```python
from build123d import *

# Parameters (mm, degrees)
BOSS_EXTRUDE1_DEPTH      = 162.5
BOSS_EXTRUDE2_DEPTH      = 43.5
BOSS_EXTRUDE2_DEPTH_BACK = 145
SKETCH3_R                = 81.25
CUT_EXTRUDE1_DEPTH       = 150
SKETCH6_R                = 87.5
SKETCH6_R_2              = 81.25
BOSS_EXTRUDE4_DEPTH      = 43.5
SKETCH7_R                = 115.75
BOSS_EXTRUDE5_DEPTH      = 12.5
SKETCH8_R                = 7.5
CUT_EXTRUDE2_DEPTH       = 12.5
CUT_EXTRUDE3_DEPTH       = 315.329842681
CUT_EXTRUDE3_DEPTH_BACK  = 315.329842681
SKETCH9_R                = 18.75


with BuildPart() as part:
    # Sketch1 → Boss-Extrude1 (new body)
    with BuildSketch(Plane.XY):
        with BuildLine():
            Line((-150, -169), (150, -169))
            Line((150, -169), (82.827141263, 28.211959701))
            ThreePointArc((82.827141263, 28.211959701), (0, 87.5), (-82.827141263, 28.211959701))
            Line((-82.827141263, 28.211959701), (-150, -169))
        make_face()
    extrude(amount=BOSS_EXTRUDE1_DEPTH)

    # Sketch2 → Boss-Extrude2 (add, two sides: drawn at the far end of the back side and taken through both)
    with BuildSketch(Plane.XY.offset(162.5).offset(-BOSS_EXTRUDE2_DEPTH_BACK)):
        with BuildLine():
            Line((-106.53243077, 150), (106.53243077, 150))
            Line((106.53243077, 150), (106.53243077, 135))
            Line((106.53243077, 135), (91.53243077, 135))
            Line((91.53243077, 135), (91.53243077, 120))
            Line((91.53243077, 120), (106.53243077, 120))
            Line((106.53243077, 120), (106.53243077, 105))
            Line((106.53243077, 105), (91.53243077, 105))
            Line((91.53243077, 105), (91.53243077, 90))
            Line((91.53243077, 90), (106.53243077, 90))
            Line((106.53243077, 90), (106.53243077, 75))
            Line((106.53243077, 75), (91.53243077, 75))
            Line((91.53243077, 75), (91.53243077, 60))
            Line((91.53243077, 60), (106.53243077, 60))
            Line((106.53243077, 60), (106.53243077, 45))
            Line((106.53243077, 45), (91.53243077, 45))
            Line((91.53243077, 45), (91.53243077, 30))
            Line((91.53243077, 30), (106.53243077, 30))
            Line((106.53243077, 30), (106.53243077, -41.384104643))
            Line((106.53243077, -41.384104643), (82.827141263, 28.211959701))
            ThreePointArc((82.827141263, 28.211959701), (0, 87.5), (-82.827141263, 28.211959701))
            Line((-82.827141263, 28.211959701), (-106.53243077, -41.384104643))
            Line((-106.53243077, -41.384104643), (-106.53243077, 30))
            Line((-106.53243077, 30), (-91.53243077, 30))
            Line((-91.53243077, 30), (-91.53243077, 45))
            Line((-91.53243077, 45), (-106.53243077, 45))
            Line((-106.53243077, 45), (-106.53243077, 60))
            Line((-106.53243077, 60), (-91.53243077, 60))
            Line((-91.53243077, 60), (-91.53243077, 75))
            Line((-91.53243077, 75), (-106.53243077, 75))
            Line((-106.53243077, 75), (-106.53243077, 90))
            Line((-106.53243077, 90), (-91.53243077, 90))
            Line((-91.53243077, 90), (-91.53243077, 105))
            Line((-91.53243077, 105), (-106.53243077, 105))
            Line((-106.53243077, 105), (-106.53243077, 120))
            Line((-106.53243077, 120), (-91.53243077, 120))
            Line((-91.53243077, 120), (-91.53243077, 135))
            Line((-91.53243077, 135), (-106.53243077, 135))
            Line((-106.53243077, 135), (-106.53243077, 150))
        make_face()
    extrude(amount=BOSS_EXTRUDE2_DEPTH + BOSS_EXTRUDE2_DEPTH_BACK)

    # Sketch3 → Cut-Extrude1 (cut)
    with BuildSketch(Plane.XY.offset(162.5)):
        Circle(SKETCH3_R)
    extrude(amount=-CUT_EXTRUDE1_DEPTH, mode=Mode.SUBTRACT)

    # Sketch6 → Boss-Extrude4 (add, through all)
    with BuildSketch(Plane.XY.offset(162.5)):
        Circle(SKETCH6_R)
        Circle(SKETCH6_R_2, mode=Mode.SUBTRACT)
    extrude(amount=BOSS_EXTRUDE4_DEPTH)

    # Sketch7 → Boss-Extrude5 (add)
    with BuildSketch(Plane.XY.offset(206)):
        with Locations(Location((0, 0, 0), (0, 0, 156.979731296))):
            Circle(SKETCH7_R)
    extrude(amount=BOSS_EXTRUDE5_DEPTH)

    # Sketch8 → Cut-Extrude2 (cut)
    with BuildSketch(Plane.XY.offset(218.5)):
        with Locations((0, -106.25)):
            Circle(SKETCH8_R)
        with Locations((-92.015199152, 53.125)):
            Circle(SKETCH8_R)
        with Locations((92.015199152, 53.125)):
            Circle(SKETCH8_R)
    extrude(amount=-CUT_EXTRUDE2_DEPTH, mode=Mode.SUBTRACT)

    # Sketch9 → Cut-Extrude3 (cut, two sides: drawn at the far end of the back side and taken through both)
    with BuildSketch(Plane.XY.offset(218.5).offset(-CUT_EXTRUDE3_DEPTH_BACK)):
        Circle(SKETCH9_R)
    extrude(amount=CUT_EXTRUDE3_DEPTH + CUT_EXTRUDE3_DEPTH_BACK, mode=Mode.SUBTRACT)


solid = part.part
```
CAD build for the part. Positions are in the model's coordinates, mm. A direction names the side the tool comes from. Round coordinates to 2 decimals unless told otherwise and drop trailing zeros. Loops run counter-clockwise (first coordinate to the right, second up) from the corner with the lowest first, then second, coordinate; pieces in that order, holes last. Notation, with made-up numbers: (9, 49.5) - (20, 49.5) arc R14 ccw to (20, 60.5) - close; hole circle Ø8 at (76, 48). An arc over 180 degrees is marked (long way). Return JSON: item names as keys, results as strings. Group by question number.
Q1. Band-saw the part on C-C on y = -106.25. Give the cut face in (x, z).
Q2. Band-saw the part on B-B on y = 0. Give the number of separate pieces and of enclosed holes in the cut face, plus the area to 3 significant figures.
Q3. Band-saw the part on A-A on x = 0. Give the cut face in (y, z).
Q4. Flat gauge pins, fed straight in: pin 1 Ø2 at (y, z) = (54, 27.5) entering from -X; pin 2 Ø12 at (y, z) = (116, 80.5) entering from +X; pin 3 Ø12 at (x, y) = (0, -106.25) entering from +Z. Where does each tip first touch, or does it go through?
Q5. Band-saw the part on D-D on y = 109.5. Give the cut face in (x, z).
Q6. Drill centre lines: line 1 along Y through (x, z) = (0, 215); line 2 along Y through (x, z) = (-102, 154); line 3 along Y through (x, z) = (0, 9.5). Where is each one in solid material? Low to high. Write a range as [from, to].
Q7. Tool access for faces 1 (the face through (99, 75, 110)), 2 (the face through (84.522, 53.455, 212.338)), 3 (the face through (-106.532, 112, 110)), 4 (the face through (106.532, -5, 110)): list every direction of +Z, -Z, +X, -X, +Y, -Y with a clear straight run to the whole face (end or side of a thin tool).
Q8. Two-plate mould, pull along Y, no slides. Class faces 5 (the face through (99, 135, 110)), 6 (the face through (-2, -169, 80)), 7 (the face through (-106.532, 142, 110)): +Y half, -Y half, draft (parallel to the pull), parting line (faces both ways), or undercut.
Solutions:
{
 "1": {"outline": "(-128.63, 0) - (128.63, 0) - (128.63, 162.5) - (-128.63, 162.5) - close; (-45.92, 206) - (-7.5, 206) - (-7.5, 218.5) - (-45.92, 218.5) - close; (7.5, 206) - (45.92, 206) - (45.92, 218.5) - (7.5, 218.5) - close"},
 "2": {"separate pieces": "2", "enclosed holes": "2", "area": "13,500 mm^2"},
 "3": {"outline": "(-169, 0) - (-18.75, 0) - (-18.75, 12.5) - (-81.25, 12.5) - (-81.25, 206) - (-18.75, 206) - (-18.75, 218.5) - (-98.75, 218.5) - (-98.75, 206) - (-87.5, 206) - (-87.5, 162.5) - (-169, 162.5) - close; (-115.75, 206) - (-113.75, 206) - (-113.75, 218.5) - (-115.75, 218.5) - close; (18.75, 0) - (87.5, 0) - (87.5, 17.5) - (150, 17.5) - (150, 206) - (115.75, 206) - (115.75, 218.5) - (18.75, 218.5) - (18.75, 206) - (81.25, 206) - (81.25, 12.5) - (18.75, 12.5) - close"},
 "4": {"pin 1": "stops at x = -106.53", "pin 2": "stops at x = 106.53", "pin 3": "stops at z = 162.5"},
 "5": {"outline": "(-106.53, 17.5) - (106.53, 17.5) - (106.53, 206) - (37.52, 206) - (37.52, 218.5) - (-37.52, 218.5) - (-37.52, 206) - (-106.53, 206) - close"},
 "6": {"line 1": "y = [-115.75, -113.75], [-98.75, -18.75], [18.75, 115.75]", "line 2": "y = [-169, 30], [45, 60], [75, 90], [105, 120], [135, 150]", "line 3": "y = [-169, -18.75], [18.75, 87.5]"},
 "7": {"face 1": "+Z, -Z, +X", "face 2": "+Z", "face 3": "+Z, -Z, -X, +Y", "face 4": "-Z, +X, +Y"},
 "8": {"face 5": "undercut", "face 6": "-Y half", "face 7": "draft"}
}
